from build123d import *

# Parameters (mm, degrees)
SKETCH1_W           = 100
SKETCH1_H           = 40
BOSS_EXTRUDE1_DEPTH = 20
SKETCH2_R           = 3
BOSS_EXTRUDE2_DEPTH = 15
SKETCH3_W           = 40
SKETCH3_H           = 40
BOSS_EXTRUDE3_DEPTH = 15


with BuildPart() as part:
    # Sketch1 → Boss-Extrude1 (new body)
    with BuildSketch(Plane(origin=(0, 0, 0), x_dir=(1, 0, 0), z_dir=(0, 1, 0))):
        with Locations((50, 20)):
            Rectangle(SKETCH1_W, SKETCH1_H)
    extrude(amount=BOSS_EXTRUDE1_DEPTH)

    # Sketch2 → Boss-Extrude2 (add)
    with BuildSketch(Plane(origin=(0, 20, 0), x_dir=(1, 0, 0), z_dir=(0, 1, 0))):
        with Locations(Location((80, 20, 0), (0, 0, 90))):
            Circle(SKETCH2_R)
    extrude(amount=BOSS_EXTRUDE2_DEPTH)

    # Sketch3 → Boss-Extrude3 (add)
    with BuildSketch(Plane(origin=(0, 20, 0), x_dir=(1, 0, 0), z_dir=(0, 1, 0))):
        with Locations((20, 20)):
            Rectangle(SKETCH3_W, SKETCH3_H)
    extrude(amount=BOSS_EXTRUDE3_DEPTH)


solid = part.part
Geometry: final body of the model. Coordinates: model frame, mm. Round coordinates to 2 decimals unless told otherwise and drop trailing zeros. Loops run counter-clockwise (first coordinate to the right, second up) from the corner with the lowest first, then second, coordinate; pieces in that order, holes last. Notation, with made-up numbers: M -14,27.5 L -3,27.5 A26 cw -3,41.5 Z; hole C 41.5,62 d7. An arc over 180 degrees is marked long. One line per question, with ' | ' between items.
(1) Cut plane D-D on z = -11. Return the cut outline in (x, y), plus the area to 3 significant figures.
Check result:
outline: M 0,0 L 100,0 L 100,20 L 40,20 L 40,35 L 0,35 Z | area: 2,600 mm2
(2) Pull-direction query (X, two-part tool) for faces 1 (the flat face through (100, 10, -20)), 2 (the cylindrical face through (82.93, 27.4, -19.35)), 3 (the flat face through (49, 0, -20)); classes: +X half, -X half, draft (parallel to the pull), parting line (faces both ways), or undercut.
Check result:
face 1: +X half | face 2: undercut | face 3: draft
(3) Cut plane C-C on y = 32. Return the cut outline in (x, z).
Check result:
outline: M 0,-40 L 40,-40 L 40,0 L 0,0 Z; C 80,-20 d6
(4) Cut plane A-A on z = -20. Return the cut outline in (x, y).
Check result:
outline: M 0,0 L 100,0 L 100,20 L 83,20 L 83,35 L 77,35 L 77,20 L 40,20 L 40,35 L 0,35 Z
(5) Material intervals for line 1 along X through (y, z) = (20.5, -4); line 2 along Y through (x, z) = (95, -26); line 3 along X through (y, z) = (33, -22.5), sorted ascending. Write a range as from..to.
Check result:
line 1: x = 0..40 | line 2: y = 0..20 | line 3: x = 0..40, 78.34..81.66
(6) Contact query for a flat-ended pin moving along its axis: P1, Ø20, axis at x = 79.5, z = -25, coming from the +Y side. Output: stop coordinate, or through.
Check result:
P1: stops at y = 35
(7) Cut plane B-B on x = 80. Return the cut outline in (y, z), plus the area to 3 significant figures.
Check result:
outline: M 0,-40 L 20,-40 L 20,-23 L 35,-23 L 35,-17 L 20,-17 L 20,0 L 0,0 Z | area: 890 mm2
